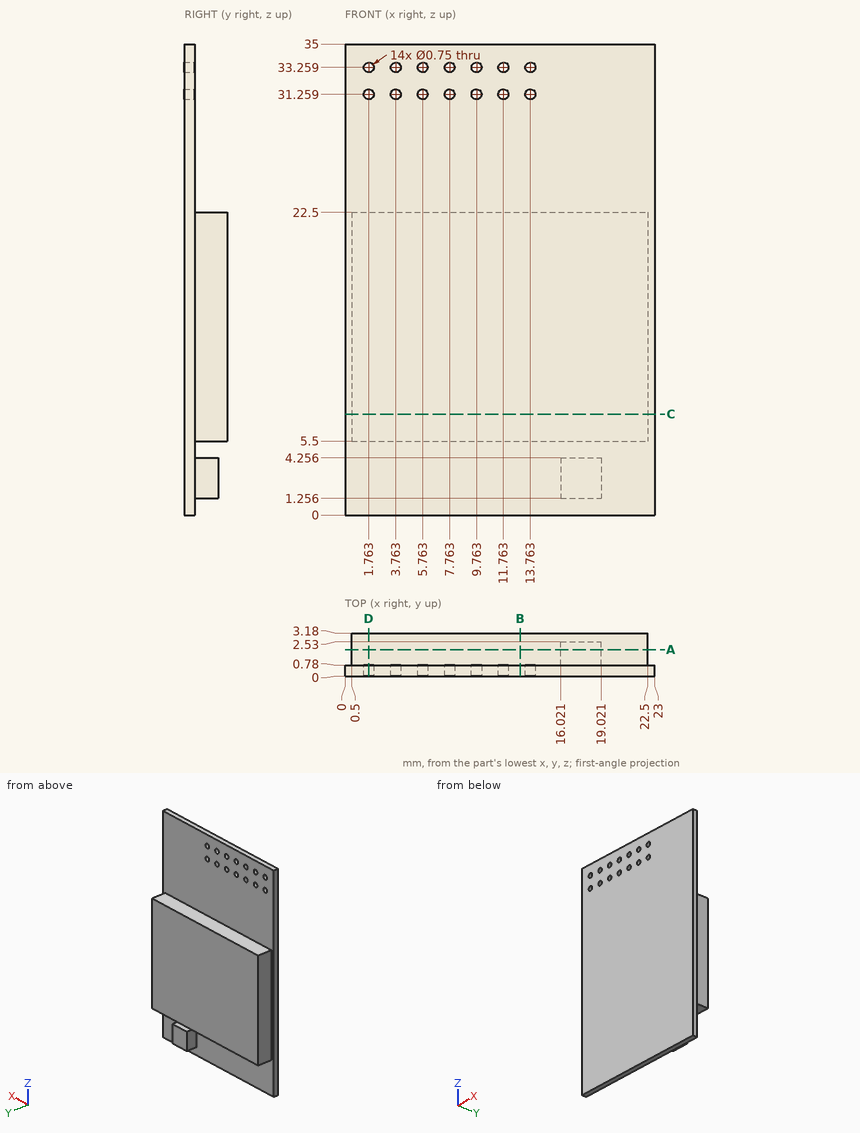
Print and shaded views of the part. All mm, measured from the part's lowest x, y and z. Coordinates: 2 decimals unless noted, no trailing zeros. Order: outer loops, then holes, each group sorted by start corner. A loop starts at its lowest first (then second) coordinate and runs counter-clockwise, first axis right, second up.
(1) Probe L1, parallel to Y at x = 21.75, z = 28; L2, parallel to X at y = 1.75, z = 19; L3, parallel to Z at x = 19.25, y = 2.8. List the from-to ranges inside material, lowest first.
Check sheet entries:
L1: y = 0 to 0.78
L2: x = 0.5 to 22.5
L3: z = 5.5 to 22.5
(2) Slice it at B-B, the plane x = 13. Write the cut outline in (y, z).
Check sheet entries:
outline: (0, 0) - (0.78, 0) - (0.78, 5.5) - (3.18, 5.5) - (3.18, 22.5) - (0.78, 22.5) - (0.78, 35) - (0, 35) - close
(3) Pin check, flat tips, straight feed: pin 1 Ø1.9 at (y, z) = (2, 3) entering from -X; pin 2 Ø0.9 at (x, y) = (18, 1.5) entering from -Z; pin 3 Ø0.7 at (x, y) = (13.5, 1.5) entering from -Z. Stop position of each tip, or through.
Check sheet entries:
pin 1: stops at x = 16.02
pin 2: stops at z = 1.26
pin 3: stops at z = 5.5
(4) Slice it at D-D, the plane x = 1.75. Write the cut outline in (y, z) (1 decimal).
Check sheet entries:
outline: (0, 0) - (0.8, 0) - (0.8, 5.5) - (3.2, 5.5) - (3.2, 22.5) - (0.8, 22.5) - (0.8, 30.9) - (0, 30.9) - close; (0, 31.6) - (0.8, 31.6) - (0.8, 32.9) - (0, 32.9) - close; (0, 33.6) - (0.8, 33.6) - (0.8, 35) - (0, 35) - close
(5) Slice it at A-A, the plane y = 1.95. Write the cut outline in (x, z).
Check sheet entries:
outline: (0.5, 5.5) - (22.5, 5.5) - (22.5, 22.5) - (0.5, 22.5) - close; (16.02, 1.26) - (19.02, 1.26) - (19.02, 4.26) - (16.02, 4.26) - close
(6) Slice it at C-C, the plane z = 7.5. Write the cut outline in (x, y).
Check sheet entries:
outline: (0, 0) - (23, 0) - (23, 0.78) - (22.5, 0.78) - (22.5, 3.18) - (0.5, 3.18) - (0.5, 0.78) - (0, 0.78) - close
